Read the model definition and answer for the solid it produces. Units are mm, in the model's axes. A direction names the side the tool comes from. Coordinates: 2 decimals unless noted, no trailing zeros. Loops run counter-clockwise (first coordinate to the right, second up) from the corner with the lowest first, then second, coordinate; pieces in that order, holes last. Notation, with made-up numbers: M -35,83 L 21,83 A19 cw 21,110 Z; hole C 16.5,-12 d8. An arc over 180 degrees is marked long. Put each result on its own line as item: value.
Autodesk Inventor part; units mm, degrees
ref_plane "YZ Plane" through (0, 0, 0) normal (1, 0, 0) x (0, 1, 0)
ref_plane "XZ Plane" through (0, 0, 0) normal (0, 1, 0) x (-1, 0, 0)
ref_plane "XY Plane" through (0, 0, 0) normal (0, 0, 1) x (1, 0, 0)
sketch "Sketch1" plane through (0, 0, 0) normal (0, 0, 1) x (1, 0, 0)
  line L0 (-23.2848, 6.1511) -> (27.5152, 6.1511)
  line L1 (27.5152, 6.1511) -> (27.5152, -6.5489)
  line L2 (27.5152, -6.5489) -> (-23.2848, -6.5489)
  line L3 (-23.2848, -6.5489) -> (-23.2848, 6.1511)
  dimension "d0" = 50.8
  dimension "d1" = 12.7
extrude "Extrusion1" add sketch "Sketch1" along normal blind 1.27
fillet "Fillet1" radius 5.08 4 edges at (-23.2848, 6.1511, 0.635) (27.5152, 6.1511, 0.635) (27.5152, -6.5489, 0.635) (-23.2848, -6.5489, 0.635)
sketch "Sketch2" plane through (0, 0, 1.27) normal (0, 0, 1) x (1, 0, 0)
  line L0 (0.8452, 4.2461) -> (9.7352, 4.2461)
  line L1 (9.7352, 4.2461) -> (9.7352, -4.6439)
  line L2 (9.7352, -4.6439) -> (0.8452, -4.6439)
  line L3 (0.8452, -4.6439) -> (0.8452, 4.2461)
  point P0 (22.4352, -6.5489)
  point P1 (27.5152, -1.4689)
  dimension "d5" = 8.89
  dimension "d6" = 17.78
  dimension "d7" = 1.905
  dimension "d8" = 8.89
extrude "Extrusion2" cut sketch "Sketch2" against normal through all
properties part number "tongue"
1) Find section A-A, the plane y = 2.25. Write down the section's boundary in (x, z), plus the area to 3 significant figures.
Answer list:
outline: M -23.15,0 L 0.85,0 L 0.85,1.27 L -23.15,1.27 Z; M 9.74,0 L 27.38,0 L 27.38,1.27 L 9.74,1.27 Z
area: 52.9 mm^2
2) Find section C-C, the plane y = -4. Write down the section's boundary in (x, z).
Answer list:
outline: M -22.61,0 L 0.85,0 L 0.85,1.27 L -22.61,1.27 Z; M 9.74,0 L 26.84,0 L 26.84,1.27 L 9.74,1.27 Z
3) Which of the six approach directions +Z, -Z, +X, -X, +Y, -Y give full straight-line access (tool end or side, diameter ignored) to faces 4 (the flat face through (5, -4.644, 1)), 5 (the flat face through (27.515, 0, 1))?
Answer list:
face 4: +Z, -Z
face 5: +Z, -Z, +X, +Y, -Y
4) Straight lines are drawn through the part: line 1 (X direction, y = 0.25, z = 0.3); line 2 (Y direction, x = 1.5, z = 1.2); line 3 (X direction, y = -2.5, z = 0.8). For each, find the intervals that lie inside material, in ascending order. Write a range as [from, to].
Answer list:
line 1: x = [-23.28, 0.85], [9.74, 27.52]
line 2: y = [-6.55, -4.64], [4.25, 6.15]
line 3: x = [-23.18, 0.85], [9.74, 27.41]
5) Determine the mould class of faces 1 (the flat face through (0.845, 0, 1)), 2 (the cylindrical face through (25.99, -5.1, 0.64)), 3 (the cylindrical face through (-21.76, 4.7, 0.64)) for opening direction X: released by +X, released by -X, zero draft, split by the parting line, or undercut.
Answer list:
face 1: undercut
face 2: released by +X
face 3: released by -X
6) Find section B-B, the plane z = 0.6. Write down the section's boundary in (x, y), plus the area to 3 significant figures.
Answer list:
outline: M -23.28,-1.47 A5.08 ccw -18.2,-6.55 L 22.44,-6.55 A5.08 ccw 27.52,-1.47 L 27.52,1.07 A5.08 ccw 22.44,6.15 L -18.2,6.15 A5.08 ccw -23.28,1.07 Z; hole M 0.85,-4.64 L 9.74,-4.64 L 9.74,4.25 L 0.85,4.25 Z
area: 544 mm^2
